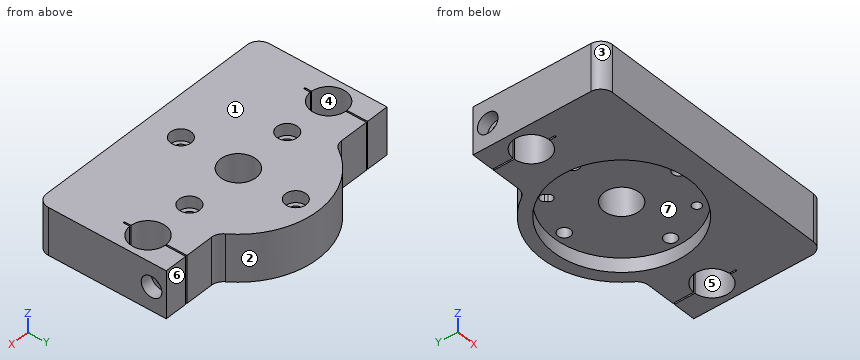
```python
from build123d import *

# Parameters (mm, degrees)
BASE_DEPTH                            = 12.7
TUBE_COUNTERBORE_D                    = 6.7564
TUBE_COUNTERBORE_CBORE_D              = 11.1125
TUBE_COUNTERBORE_CBORE_DEPTH          = 6.35
TUBE_COUNTERBORE_PATTERN_COUNT        = 4
SKETCH8_R                             = 36.5125
STRUCTURE_TUBE_RECESS_DEPTH           = 7.62
SKETCH9_R                             = 9.525
LEAD_SCREW_THRU_HOLE_DEPTH            = 88.275546726
SKETCH13_R                            = 9.525
RAIL_BORE_PILOT_HOLE_DEPTH            = 90.140634148
SKETCH14_R                            = 2.38125
ALIGNMENT_FEATURES_DEPTH              = 6.35
GENERIC_ROUNDING_FILLET_R             = 6.35
SKETCH15_W                            = 0.79375
SKETCH15_H                            = 11.120771821
FLEXURE_SLITS_DEPTH                   = 90.140634148
FLEXURE_CLAMP_COUNTERBORE_D           = 6.7564
FLEXURE_CLAMP_COUNTERBORE_DEPTH       = 12.303125
FLEXURE_CLAMP_COUNTERBORE_CBORE_D     = 11.1125
FLEXURE_CLAMP_COUNTERBORE_CBORE_DEPTH = 6.35


with BuildPart() as part:
    # Bolt circle → Base (new, symmetric)
    with BuildSketch(Plane.XY):
        with BuildLine():
            Line((37.567106623, 20.6375), (69.85, 20.6375))
            Line((69.85, 20.6375), (69.85, -49.2125))
            Line((69.85, -49.2125), (-69.85, -49.2125))
            Line((-69.85, -49.2125), (-69.85, 20.6375))
            Line((-69.85, 20.6375), (-37.567106623, 20.6375))
            ThreePointArc((-37.567106623, 20.6375), (0, 42.8625), (37.567106623, 20.6375))
        make_face()
    extrude(amount=BASE_DEPTH, both=True)

    # Tube counterbore (through all)
    with Locations(Plane.XY.offset(12.7)):
        with Locations((0, 30.95625)):
            tube_counterbore = CounterBoreHole(TUBE_COUNTERBORE_D / 2, TUBE_COUNTERBORE_CBORE_D / 2, TUBE_COUNTERBORE_CBORE_DEPTH)

    # Tube counterbore pattern: Tube counterbore ×4 about axis
    tube_counterbore_pattern_axis = Axis((0, 0, 0), (0, 0, 1))
    for i in range(1, TUBE_COUNTERBORE_PATTERN_COUNT):
        add(tube_counterbore.rotate(tube_counterbore_pattern_axis, i * 360 / TUBE_COUNTERBORE_PATTERN_COUNT), mode=Mode.SUBTRACT)

    # Sketch8 → Structure_tube_recess (cut)
    with BuildSketch(Plane(origin=(0, 0, -12.7), x_dir=(-1, 0, 0), z_dir=(0, 0, -1))):
        Circle(SKETCH8_R)
    extrude(amount=-STRUCTURE_TUBE_RECESS_DEPTH, mode=Mode.SUBTRACT)

    # Sketch9 → Lead_screw_thru_hole (cut, through all)
    with BuildSketch(Plane(origin=(0, 0, -5.08), x_dir=(-1, 0, 0), z_dir=(0, 0, -1))):
        Circle(SKETCH9_R)
    extrude(amount=-LEAD_SCREW_THRU_HOLE_DEPTH, mode=Mode.SUBTRACT)

    # Sketch13 → Rail_bore_pilot_hole (cut, through all)
    with BuildSketch(Plane.XY.offset(12.7)):
        with Locations((57.15, 0)):
            Circle(SKETCH13_R)
        with Locations((-57.15, 0)):
            Circle(SKETCH13_R)
    extrude(amount=-RAIL_BORE_PILOT_HOLE_DEPTH, mode=Mode.SUBTRACT)

    # Sketch14 → Alignment_features (cut)
    with BuildSketch(Plane(origin=(0, 0, -5.08), x_dir=(-1, 0, 0), z_dir=(0, 0, -1))):
        with Locations((-21.889374295, -21.889374295)):
            Circle(SKETCH14_R)
        with BuildLine():
            Line((20.681324246, 24.089602852), (19.602797121, 22.924727111))
            ThreePointArc((19.602797121, 22.924727111), (19.732320046, 19.559622813), (23.097424344, 19.689145738))
            Line((23.097424344, 19.689145738), (24.175951469, 20.854021479))
            ThreePointArc((24.175951469, 20.854021479), (24.046428544, 24.219125777), (20.681324246, 24.089602852))
        make_face()
    extrude(amount=-ALIGNMENT_FEATURES_DEPTH, mode=Mode.SUBTRACT)

    # Generic_rounding_fillet
    generic_rounding_fillet_edges = [part.edges().sort_by_distance(p)[0] for p in [
        (37.567106623, 20.6375, 0),
        (69.85, -49.2125, 0),
        (-69.85, -49.2125, 0),
        (-37.567106623, 20.6375, 0),
    ]]
    fillet(generic_rounding_fillet_edges, radius=GENERIC_ROUNDING_FILLET_R)

    # Sketch15 → Flexure_slits (cut, through all)
    with BuildSketch(Plane(origin=(0, 0, -12.7), x_dir=(-1, 0, 0), z_dir=(0, 0, -1))):
        with BuildLine():
            Line((56.753125, -9.516728179), (56.753125, -12.7))
            ThreePointArc((56.753125, -12.7), (57.15, -13.096875), (57.546875, -12.7))
            Line((57.546875, -12.7), (57.546875, -9.516728179))
            ThreePointArc((57.546875, -9.516728179), (57.15, -9.525), (56.753125, -9.516728179))
        make_face()
        with Locations((57.15, 15.07711409)):
            Rectangle(SKETCH15_W, SKETCH15_H)
        with BuildLine():
            Line((-57.546875, -12.7), (-57.546875, -9.516728179))
            ThreePointArc((-57.546875, -9.516728179), (-57.15, -9.525), (-56.753125, -9.516728179))
            Line((-56.753125, -9.516728179), (-56.753125, -12.7))
            ThreePointArc((-56.753125, -12.7), (-57.15, -13.096875), (-57.546875, -12.7))
        make_face()
        with Locations((-57.15, 15.07711409)):
            Rectangle(SKETCH15_W, SKETCH15_H)
    extrude(amount=-FLEXURE_SLITS_DEPTH, mode=Mode.SUBTRACT)

    # Flexure_clamp_counterbore
    with Locations(Plane(origin=(-69.85, 5.772256362, 0.258118138), x_dir=(0, 0, 1), z_dir=(-1, 0, 0))):
        with Locations((-0.258118138, 6.927743638)):
            flexure_clamp_counterbore = CounterBoreHole(FLEXURE_CLAMP_COUNTERBORE_D / 2, FLEXURE_CLAMP_COUNTERBORE_CBORE_D / 2, FLEXURE_CLAMP_COUNTERBORE_CBORE_DEPTH, depth=FLEXURE_CLAMP_COUNTERBORE_DEPTH)

    # Sketch18 → Flexure_clamp_threads (revolve, cut)
    with BuildSketch(Plane(origin=(-56.753125, 12.7, 0), x_dir=(0, 0, 1), z_dir=(0, 1, 0))):
        Polygon((0, 0), (0, 18.043816902), (2.5527, 16.51), (2.5527, 0), align=None)
    flexure_clamp_threads = revolve(axis=Axis((-63.103125, 12.7, 0), (1, 0, 0)), mode=Mode.SUBTRACT)

    # Flexure_clamp_fastener_holes: Flexure_clamp_counterbore, Flexure_clamp_threads across plane
    add(flexure_clamp_counterbore.mirror(Plane(origin=(0, 0, 0), x_dir=(0, 0, 1), z_dir=(1, 0, 0))), mode=Mode.SUBTRACT)
    add(flexure_clamp_threads.mirror(Plane(origin=(0, 0, 0), x_dir=(0, 0, 1), z_dir=(1, 0, 0))), mode=Mode.SUBTRACT)


solid = part.part
```
Geometry check sheet. Reference: the model listing, model coordinates, mm. Face numbers are marked on the shaded views. A direction names the side the tool comes from. Round coordinates to 2 decimals unless told otherwise and drop trailing zeros. Order: outer loops, then holes, each group sorted by start corner. A loop starts at its lowest first (then second) coordinate and runs counter-clockwise, first axis right, second up. Notation, with made-up numbers: (27, -23) -> (33, -23) arc R20 ccw to (33, -16) -> close; hole circle Ø6 at (-3, -2.5). An arc over 180 degrees is marked (long way). Return JSON: item names as keys, results as strings. Group by question number.
Q1. Tool access check on the marked faces 5, 6 and 7. Record the directions out of +Z, -Z, +X, -X, +Y, -Y that give a thin tool (end or side, any length) a straight path to the whole face; none if there is none.
Q2. Gauge pin test, flat ends, axial feed: pin 1 (1.8 mm diameter, centred on x = -21.5, y = 23, fed in from -Z); pin 2 (5 mm diameter, centred on x = -29, y = 10, fed in from -Z); pin 3 (4.5 mm diameter, centred on x = 49.5, z = 4, fed in from +Y); pin 4 (4 mm diameter, centred on x = 30.96, y = 0, fed in from -Z). Record the tip position at first contact, or that the pin passes through.
Q3. Material ranges on probe 1 along Y at (x, z) = (0, 10.25) (1 decimal); probe 2 along Y at (x, z) = (0, 2.5) (1 decimal); probe 3 along Y at (x, z) = (-44.75, 0), recorded low to high. Write a range as from..to.
Q4. Section check D-D, the plane x = 29. Record the boundary of the cut face in (y, z), plus the area to 3 significant figures.
Q5. Release check for a two-part mould opening along Y. For the marked faces 1, 2, 3 and 4 record: released by +Y, released by -Y, zero draft, split by the parting line, or undercut.
Q6. Section check B-B, the plane x = 0. Count the separate pieces of the cut face and the enclosed holes in it, plus the area to 3 significant figures.
Numbers:
{
 "1": {"face 5": "+Z, -Z", "face 6": "+Z, -Z, +X, +Y", "face 7": "-Z"},
 "2": {"pin 1": "z = 1.27", "pin 2": "z = -5.08", "pin 3": "y = 20.64", "pin 4": "through"},
 "3": {"probe 1": "-49.2..-36.5, -25.4..-9.5, 9.5..25.4, 36.5..42.9", "probe 2": "-49.2..-34.3, -27.6..-9.5, 9.5..27.6, 34.3..42.9", "probe 3": "-49.21..10.15, 15.25..20.64"},
 "4": {"outline": "(-49.21, -12.7) -> (-22.18, -12.7) -> (-22.18, -5.08) -> (-2.75, -5.08) -> (-2.75, 6.35) -> (-5.2, 6.35) -> (-5.2, 12.7) -> (-49.21, 12.7) -> close; (2.75, -5.08) -> (22.18, -5.08) -> (22.18, -12.7) -> (31.56, -12.7) -> (31.56, 12.7) -> (5.2, 12.7) -> (5.2, 6.35) -> (2.75, 6.35) -> close", "area": "1,580 mm^2"},
 "5": {"face 1": "zero draft", "face 2": "released by +Y", "face 3": "released by -Y", "face 4": "undercut"},
 "6": {"separate pieces": "4", "enclosed holes": "0", "area": "1,150 mm^2"}
}
